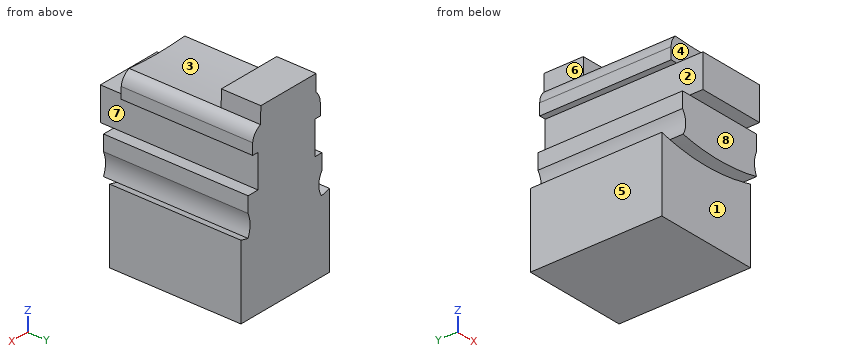
```python
from build123d import *

# Parameters (mm, degrees)
F1_DEPTH = 25.4
F2_DEPTH = 27.94
F0_W     = 12.805208
F0_H     = 6.38972
F3_DEPTH = 30.48
F4_DEPTH = 25.4
F5_DEPTH = 7.62


with BuildPart() as f1:
    # F0 (on Front) → F1 (new body)
    with BuildSketch(Plane.XZ):
        with BuildLine():
            Line((-20.041954, 0), (0, 0))
            Line((0, 0), (0, 14.202959))
            ThreePointArc((0, 14.202959), (-0.809395, 13.992635), (-1.623196, 13.800062))
            ThreePointArc((-1.623196, 13.800062), (-9.906257, 12.866678), (-18.194769, 13.750344))
            ThreePointArc((-18.194769, 13.750344), (-19.121176, 13.965165), (-20.041954, 14.202959))
            Line((-20.041954, 14.202959), (-20.041954, 0))
        make_face()
    extrude(amount=F1_DEPTH)

    # F0 (on Front) → F2 (join)
    with BuildSketch(Plane.XZ):
        with BuildLine():
            ThreePointArc((-18.194769, 13.750344), (-9.906257, 12.866678), (-1.623196, 13.800062))
            ThreePointArc((-1.623196, 13.800062), (-2.065342, 15.917783), (-1.623196, 18.035505))
            Line((-1.623196, 18.035505), (-1.623196, 21.024244))
            Line((-1.623196, 21.024244), (-3.877633, 21.024244))
            Line((-3.877633, 21.024244), (-16.682841, 21.024244))
            Line((-16.682841, 21.024244), (-18.318918, 21.024244))
            Line((-18.318918, 21.024244), (-18.318918, 18.035505))
            ThreePointArc((-18.318918, 18.035505), (-17.605755, 15.911787), (-18.194769, 13.750344))
        make_face()
    extrude(amount=F2_DEPTH)

    # F0 (on Front) → F3 (join)
    with BuildSketch(Plane.XZ):
        with Locations((-10.280237, 24.219104)):
            Rectangle(F0_W, F0_H)
    extrude(amount=F3_DEPTH)

    # F0 (on Front) → F4 (join)
    with BuildSketch(Plane.XZ):
        with BuildLine():
            Line((-16.682841, 27.413964), (-3.877633, 27.413964))
            Line((-3.877633, 27.413964), (-2.653796, 27.413964))
            Line((-2.653796, 27.413964), (-2.653796, 29.587325))
            ThreePointArc((-2.653796, 29.587325), (-3.230513, 30.973826), (-4.442622, 31.860266))
            ThreePointArc((-4.442622, 31.860266), (-10.714561, 31.576369), (-16.986499, 31.860266))
            ThreePointArc((-16.986499, 31.860266), (-17.681629, 30.842499), (-17.938741, 29.637115))
            Line((-17.938741, 29.637115), (-17.938741, 27.413964))
            Line((-17.938741, 27.413964), (-16.682841, 27.413964))
        make_face()
    extrude(amount=F4_DEPTH)

    # F0 (on Front) → F5 (join)
    with BuildSketch(Plane.XZ):
        with BuildLine():
            ThreePointArc((-16.986499, 31.860266), (-10.714561, 31.576369), (-4.442622, 31.860266))
            Line((-4.442622, 31.860266), (-4.501514, 35.040405))
            Line((-4.501514, 35.040405), (-16.986499, 35.040405))
            Line((-16.986499, 35.040405), (-16.986499, 34.039252))
            Line((-16.986499, 34.039252), (-16.986499, 31.860266))
        make_face()
    extrude(amount=F5_DEPTH)


solid = f1.part
```
Build history of the part. All positions in model axes, mm. Face numbers are marked on the shaded views. A direction names the side the tool comes from. Round coordinates to 2 decimals unless told otherwise and drop trailing zeros. Loops run counter-clockwise (first coordinate to the right, second up) from the corner with the lowest first, then second, coordinate; pieces in that order, holes last. Notation, with made-up numbers: M 1,-29.5 L 34,-29.5 A24 ccw 34,-3.5 Z; hole C -22.5,4 d5. An arc over 180 degrees is marked long. Answer as CSV lines item,"result".
1. Two-plate mould, pull along X, no slides. Class the marked faces 1, 2 and 3: released by +X, released by -X, zero draft, split by the parting line, or undercut.
Resolved:
face 1,"zero draft"
face 2,"released by -X"
face 3,"undercut"
2. Cut at B-B on x = -11. Write the cut outline in (y, z).
Resolved:
outline,"M -30.48,21.02 L -27.94,21.02 L -27.94,12.88 L -25.4,12.88 L -25.4,0 L 0,0 L 0,35.04 L -7.62,35.04 L -7.62,31.58 L -25.4,31.58 L -25.4,27.41 L -30.48,27.41 Z"
3. Cut at D-D on z = 3.5. Write the cut outline in (x, y).
Resolved:
outline,"M -20.04,-25.4 L 0,-25.4 L 0,0 L -20.04,0 Z"
4. Flat gauge pins, fed straight in: P1, Ø2.5, axis at y = -12.5, z = 19.5, coming from the +X side; P2, Ø2.5, axis at x = -3, y = -15.5, coming from the +Z side; P3, Ø5, axis at y = -27.5, z = 30.5, coming from the +X side. Where does each tip first touch, or does it go through?
Resolved:
P1,"stops at x = -1.62"
P2,"stops at z = 31.78"
P3,"stops at x = -2.65"
5. Cut at A-A on y = -7. Write the cut outline in (x, z).
Resolved:
outline,"M -20.04,0 L 0,0 L 0,14.2 A38.24 cw -1.62,13.8 A5.29 cw -1.62,18.04 L -1.62,21.02 L -3.88,21.02 L -3.88,27.41 L -2.65,27.41 L -2.65,29.59 A2.79 ccw -4.44,31.86 L -4.5,35.04 L -16.99,35.04 L -16.99,31.86 A3.19 ccw -17.94,29.64 L -17.94,27.41 L -16.68,27.41 L -16.68,21.02 L -18.32,21.02 L -18.32,18.04 A3.85 cw -18.19,13.75 A38.24 cw -20.04,14.2 Z"
6. Wall check: probe 1 along X at (y, z) = (-21.5, 23); probe 2 along Y at (x, z) = (-18.25, 10.5); probe 3 along Y at (x, z) = (-13.5, 32.5). Give the ranges that are in metal, low to high. Write a range as [from, to].
Resolved:
probe 1,"x = [-16.68, -3.88]"
probe 2,"y = [-25.4, 0]"
probe 3,"y = [-7.62, 0]"
7. 3-axis set-ups, long thin cutter, end or side, ignore diameter. For the marked faces 4, 5, 6, 7 and 8: which of +Z, -Z, +X, -X, +Y, -Y reach the whole face in a straight line?
Resolved:
face 4,"+Z, +X, -X, -Y"
face 5,"+Z, -Z, -X, +Y, -Y"
face 6,"+Z, -X, +Y, -Y"
face 7,"+X, +Y, -Y"
face 8,"-Z, +X, -X, -Y"
8. Cut at C-C on y = -18. Write the cut outline in (x, z), then the cut area to 3 significant figures.
Resolved:
outline,"M -20.04,0 L 0,0 L 0,14.2 A38.24 cw -1.62,13.8 A5.29 cw -1.62,18.04 L -1.62,21.02 L -3.88,21.02 L -3.88,27.41 L -2.65,27.41 L -2.65,29.59 A2.79 ccw -4.44,31.86 A69.42 cw -16.99,31.86 A3.19 ccw -17.94,29.64 L -17.94,27.41 L -16.68,27.41 L -16.68,21.02 L -18.32,21.02 L -18.32,18.04 A3.85 cw -18.19,13.75 A38.24 cw -20.04,14.2 Z"
area,"540 mm²"
